The drawing under review shows one solid part. Ordinate dimensions are in mm from its lowest x, y, z. A direction names the side the tool comes from. Round coordinates to 2 decimals unless told otherwise and drop trailing zeros. Order: outer loops, then holes, each group sorted by start corner. A loop starts at its lowest first (then second) coordinate and runs counter-clockwise, first axis right, second up. Notation, with made-up numbers: M -17.75,56.25 L 10.25,56.25 A21 ccw 10.25,87.25 Z; hole C 67.5,-27 d3. An arc over 180 degrees is marked long. Answer as a JSON object with one key per item and string values. Group by question number.
1) To check wall thickness, follow line 1 (X direction, y = 4.5, z = 2); line 2 (X direction, y = 7.5, z = 6); line 3 (Z direction, x = 40.5, y = 50.5). State the ranges of each line that lie inside material, in increasing order.
2) Insertion check: pin 1 Ø11 at (y, z) = (5, 11.5) entering from -X; pin 2 Ø3 at (x, y) = (45.5, 4.5) entering from +Z; pin 3 Ø8 at (x, z) = (14, 12.5) entering from -Y. Each pin has a flat end and moves straight along its axis. Give the tip position at first contact, or say it passes through.
3) Consider section A-A, the plane x = 23.5. Write out the cut boundary in (y, z), then the cut area to 3 significant figures.
4) Consider section B-B, the plane z = 12.5. Write out the cut boundary in (x, y), then the cut area to 3 significant figures.
5) Consider section C-C, the plane x = 56. Write out the cut boundary in (y, z), then the cut area to 3 significant figures.
6) Consider section D-D, the plane y = 43.5. Write out the cut boundary in (x, z).
7) For the marked faces 1, 2, 3 and 4, list the 3-axis set-ups (+Z, -Z, +X, -X, +Y, -Y) from which the entire face can be reached by the end or side of a thin tool; tool diameter is ignored.
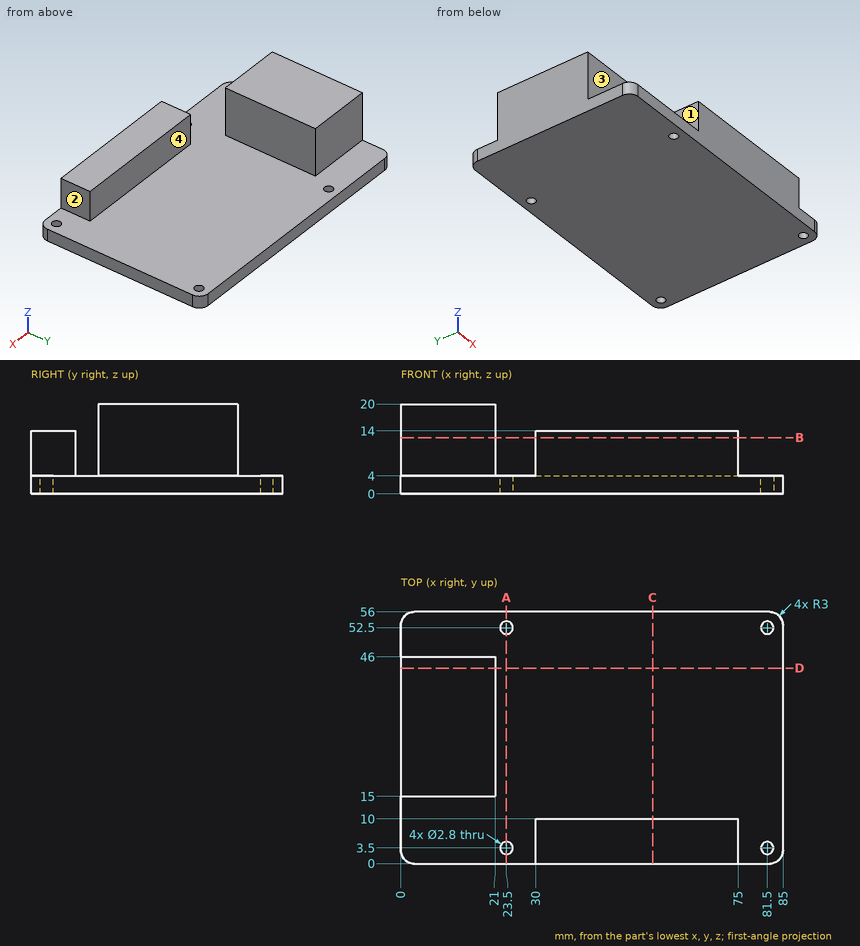
Results list:
{
 "1": {"line 1": "0 to 22.52, 24.48 to 80.52, 82.48 to 85", "line 2": "30 to 75", "line 3": "0 to 4"},
 "2": {"pin 1": "x = 30", "pin 2": "z = 14", "pin 3": "y = 15"},
 "3": {"outline": "M 0,0 L 2.1,0 L 2.1,4 L 0,4 Z; M 4.9,0 L 51.1,0 L 51.1,4 L 4.9,4 Z; M 53.9,0 L 56,0 L 56,4 L 53.9,4 Z", "area": "202 mm^2"},
 "4": {"outline": "M 0,15 L 21,15 L 21,46 L 0,46 Z; M 30,0 L 75,0 L 75,10 L 30,10 Z", "area": "1,100 mm^2"},
 "5": {"outline": "M 0,0 L 56,0 L 56,4 L 10,4 L 10,14 L 0,14 Z", "area": "324 mm^2"},
 "6": {"outline": "M 0,0 L 85,0 L 85,4 L 21,4 L 21,20 L 0,20 Z"},
 "7": {"face 1": "+Z, -X, +Y, -Y", "face 2": "+Z, +X, +Y, -Y", "face 3": "+Z, +X, -X, -Y", "face 4": "+Z, +X, -X, +Y"}
}
